Source: CAD feature listing. Evaluate the final solid. Frame: model axes, mm. Face numbers are marked on the shaded views. A direction names the side the tool comes from. Round coordinates to 2 decimals unless told otherwise and drop trailing zeros. Loops run counter-clockwise (first coordinate to the right, second up) from the corner with the lowest first, then second, coordinate; pieces in that order, holes last. Notation, with made-up numbers: M -38.75,37.25 L -4.75,37.25 A20 cw -4.75,43.25 Z; hole C 74,65 d2. An arc over 180 degrees is marked long. Answer as CSV lines item,"result". Start each with the question number.
```python
from build123d import *

# Parameters (mm, degrees)
F1_DEPTH       = 38.1
F2_T           = -7.62
F3_R           = 7.62
F4_DEPTH       = 30.48
F6_DEPTH       = 4.572
F8_D           = 6.858
F8_CBORE_D     = 12.7
F8_CBORE_DEPTH = 6.35


with BuildPart() as f1:
    # F0 (on Top) → F1 (new body)
    with BuildSketch(Plane.XY):
        with BuildLine():
            ThreePointArc((0, 12.7), (3.7197438789, 3.7197438789), (12.7, 0))
            Line((12.7, 0), (190.5, 0))
            ThreePointArc((190.5, 0), (199.4802561211, 3.7197438789), (203.2, 12.7))
            Line((203.2, 12.7), (203.2, 44.45))
            Line((203.2, 44.45), (203.2, 76.2))
            ThreePointArc((203.2, 76.2), (199.4802561211, 85.1802561211), (190.5, 88.9))
            Line((190.5, 88.9), (12.7, 88.9))
            ThreePointArc((12.7, 88.9), (3.7197438789, 85.1802561211), (0, 76.2))
            Line((0, 76.2), (0, 44.45))
            Line((0, 44.45), (0, 12.7))
        make_face()
    extrude(amount=F1_DEPTH)

    # F2
    f2_openings = [f1.faces().sort_by_distance(p)[0] for p in [
        (101.6, 44.45, 38.1),
    ]]
    offset(amount=F2_T, openings=f2_openings)

    # F3 (on face) → F4 (join, through all)
    with BuildSketch(Plane.XY.offset(38.1)):
        with Locations((9.1078975516, 79.7921024484)):
            Circle(F3_R)
        with Locations((194.0921024484, 79.7921024484)):
            Circle(F3_R)
        with Locations((9.1078975516, 9.1078975516)):
            Circle(F3_R)
        with Locations((194.0921024484, 9.1078975516)):
            Circle(F3_R)
    extrude(amount=-F4_DEPTH)

    # F5 (on face) → F6 (join)
    with BuildSketch(Plane.XY.offset(38.1)):
        with BuildLine():
            ThreePointArc((14.2957024402, 83.82), (11.9960162975, 85.6909199873), (9.1078975516, 86.36))
            Line((9.1078975516, 86.36), (9.1078975516, 83.82))
            ThreePointArc((9.1078975516, 83.82), (11.9560512242, 82.6402561211), (13.1357951031, 79.7921024484))
            ThreePointArc((13.1357951031, 79.7921024484), (9.1078975516, 75.7642048969), (5.08, 79.7921024484))
            Line((5.08, 79.7921024484), (2.54, 79.7921024484))
            ThreePointArc((2.54, 79.7921024484), (3.2090800127, 76.9039837025), (5.08, 74.6042975598))
            ThreePointArc((5.08, 74.6042975598), (11.9960162975, 73.8932849095), (15.6757951031, 79.7921024484))
            ThreePointArc((15.6757951031, 79.7921024484), (15.3211997844, 81.9209879811), (14.2957024402, 83.82))
        make_face()
        with BuildLine():
            Line((194.0921024484, 86.36), (101.6, 86.36))
            Line((101.6, 86.36), (9.1078975516, 86.36))
            ThreePointArc((9.1078975516, 86.36), (11.9960162975, 85.6909199873), (14.2957024402, 83.82))
            Line((14.2957024402, 83.82), (101.6, 83.82))
            Line((101.6, 83.82), (188.9042975598, 83.82))
            ThreePointArc((188.9042975598, 83.82), (191.2039837025, 85.6909199873), (194.0921024484, 86.36))
        make_face()
        with BuildLine():
            Line((194.0921024484, 83.82), (194.0921024484, 86.36))
            ThreePointArc((194.0921024484, 86.36), (191.2039837025, 85.6909199873), (188.9042975598, 83.82))
            ThreePointArc((188.9042975598, 83.82), (189.4478975516, 75.1478975516), (198.12, 74.6042975598))
            ThreePointArc((198.12, 74.6042975598), (199.9909199873, 76.9039837025), (200.66, 79.7921024484))
            Line((200.66, 79.7921024484), (198.12, 79.7921024484))
            ThreePointArc((198.12, 79.7921024484), (191.2439487758, 76.9439487758), (194.0921024484, 83.82))
        make_face()
        with BuildLine():
            Line((200.66, 44.45), (200.66, 79.7921024484))
            ThreePointArc((200.66, 79.7921024484), (199.9909199873, 76.9039837025), (198.12, 74.6042975598))
            Line((198.12, 74.6042975598), (198.12, 44.45))
            Line((198.12, 44.45), (198.12, 14.2957024402))
            ThreePointArc((198.12, 14.2957024402), (199.9909199873, 11.9960162975), (200.66, 9.1078975516))
            Line((200.66, 9.1078975516), (200.66, 44.45))
        make_face()
        with BuildLine():
            Line((198.12, 9.1078975516), (200.66, 9.1078975516))
            ThreePointArc((200.66, 9.1078975516), (199.9909199873, 11.9960162975), (198.12, 14.2957024402))
            ThreePointArc((198.12, 14.2957024402), (189.4478975516, 13.7521024484), (188.9042975598, 5.08))
            ThreePointArc((188.9042975598, 5.08), (191.2039837025, 3.2090800127), (194.0921024484, 2.54))
            Line((194.0921024484, 2.54), (194.0921024484, 5.08))
            ThreePointArc((194.0921024484, 5.08), (191.2439487758, 11.9560512242), (198.12, 9.1078975516))
        make_face()
        with BuildLine():
            Line((101.6, 2.54), (194.0921024484, 2.54))
            ThreePointArc((194.0921024484, 2.54), (191.2039837025, 3.2090800127), (188.9042975598, 5.08))
            Line((188.9042975598, 5.08), (101.6, 5.08))
            Line((101.6, 5.08), (14.2957024402, 5.08))
            ThreePointArc((14.2957024402, 5.08), (11.9960162975, 3.2090800127), (9.1078975516, 2.54))
            Line((9.1078975516, 2.54), (101.6, 2.54))
        make_face()
        with BuildLine():
            ThreePointArc((5.08, 14.2957024402), (3.2090800127, 11.9960162975), (2.54, 9.1078975516))
            Line((2.54, 9.1078975516), (5.08, 9.1078975516))
            ThreePointArc((5.08, 9.1078975516), (9.1078975516, 13.1357951031), (13.1357951031, 9.1078975516))
            ThreePointArc((13.1357951031, 9.1078975516), (11.9560512242, 6.2597438789), (9.1078975516, 5.08))
            Line((9.1078975516, 5.08), (9.1078975516, 2.54))
            ThreePointArc((9.1078975516, 2.54), (11.9960162975, 3.2090800127), (14.2957024402, 5.08))
            ThreePointArc((14.2957024402, 5.08), (15.3211997844, 6.9790120189), (15.6757951031, 9.1078975516))
            ThreePointArc((15.6757951031, 9.1078975516), (11.9960162975, 15.0067150905), (5.08, 14.2957024402))
        make_face()
        with BuildLine():
            ThreePointArc((5.08, 74.6042975598), (3.2090800127, 76.9039837025), (2.54, 79.7921024484))
            Line((2.54, 79.7921024484), (2.54, 44.45))
            Line((2.54, 44.45), (2.54, 9.1078975516))
            ThreePointArc((2.54, 9.1078975516), (3.2090800127, 11.9960162975), (5.08, 14.2957024402))
            Line((5.08, 14.2957024402), (5.08, 44.45))
            Line((5.08, 44.45), (5.08, 74.6042975598))
        make_face()
    extrude(amount=F6_DEPTH)

    # F8 (through all)
    with Locations(Plane(origin=(0, 0, 0), x_dir=(1, 0, 0), z_dir=(0, 0, -1))):
        with Locations((194.0921024484, -79.7921024484), (194.0921024484, -9.1078975516), (9.1078975516, -9.1078975516), (9.1078975516, -79.7921024484)):
            CounterBoreHole(F8_D / 2, F8_CBORE_D / 2, F8_CBORE_DEPTH)


solid = f1.part
```
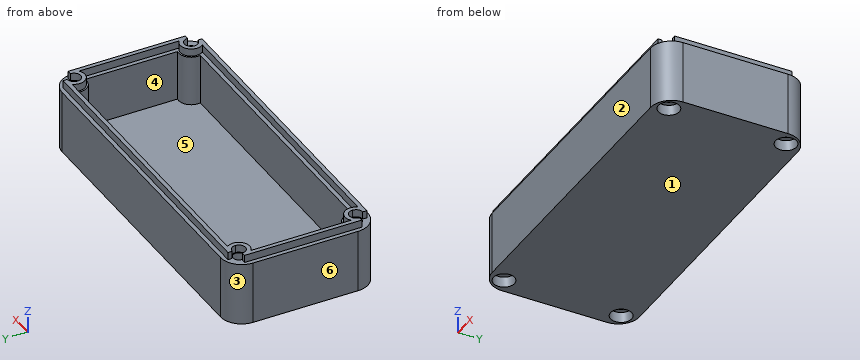
1) Contact query for flat-ended pins moving along their axis: pin 1 Ø2.5 at (x, z) = (95, 40) entering from -Y; pin 2 Ø3 at (x, y) = (29.5, 79) entering from -Z; pin 3 Ø3.5 at (y, z) = (47, 41.5) entering from +X; pin 4 Ø2 at (x, y) = (152, 30) entering from +Z. Output: stop coordinate, or through.
2) Access query for the marked faces 5 and 6. Directions: +Z, -Z, +X, -X, +Y, -Y. A direction counts if a zero-diameter tool reaches every point of the face in a straight line with its end or side. Return the directions, or none.
3) Section B-B, the plane y = 51.5. Return loops of the section in (x, z), and give its area (3 significant figures).
4) Section A-A, the plane z = 4. Return loops of the section in (x, y).
5) Ray query, line 1 along X through (y, z) = (50, 23); line 2 along Y through (x, z) = (28.5, 40); line 3 along Y through (x, z) = (149, 36.5). Return the intervals inside material, ascending.
6) Section C-C, the plane x = 26.5. Return loops of the section in (y, z).
7) Mould query, pull axis Y, two halves, no side actions, for the marked faces 1, 2, 3 and 4. Classes: pulls with the +Y half, pulls with the -Y half, needs draft (parallel to the pull), parting line crosses it, or undercut.
Findings below:
1,pin 1,"y = 2.54"
1,pin 2,"z = 0"
1,pin 3,"x = 200.66"
1,pin 4,"z = 7.62"
2,face 5,"+Z"
2,face 6,"+Z, -Z, -X, +Y, -Y"
3,outline,"M 0,0 L 203.2,0 L 203.2,38.1 L 200.66,38.1 L 200.66,42.67 L 198.12,42.67 L 198.12,38.1 L 195.58,38.1 L 195.58,7.62 L 7.62,7.62 L 7.62,38.1 L 5.08,38.1 L 5.08,42.67 L 2.54,42.67 L 2.54,38.1 L 0,38.1 Z"
3,area,"2,040 mm²"
4,outline,"M 0,12.7 A12.7 ccw 12.7,0 L 190.5,0 A12.7 ccw 203.2,12.7 L 203.2,76.2 A12.7 ccw 190.5,88.9 L 12.7,88.9 A12.7 ccw 0,76.2 Z; hole C 9.11,9.11 d12.7; hole C 9.11,79.79 d12.7; hole C 194.09,9.11 d12.7; hole C 194.09,79.79 d12.7"
5,line 1,"0 to 7.62, 195.58 to 203.2"
5,line 2,"2.54 to 5.08, 83.82 to 86.36"
5,line 3,"0 to 7.62, 81.28 to 88.9"
6,outline,"M 0,0 L 88.9,0 L 88.9,38.1 L 86.36,38.1 L 86.36,42.67 L 83.82,42.67 L 83.82,38.1 L 81.28,38.1 L 81.28,7.62 L 7.62,7.62 L 7.62,38.1 L 5.08,38.1 L 5.08,42.67 L 2.54,42.67 L 2.54,38.1 L 0,38.1 Z"
7,face 1,"needs draft"
7,face 2,"pulls with the -Y half"
7,face 3,"pulls with the +Y half"
7,face 4,"undercut"
